from build123d import *

# Parameters (mm, degrees)
F2_R     = 1.5728770132
F3_DEPTH = 20.955
F4_R     = 4.7463390005
F5_DEPTH = 9.525


# Not quite as in the source:
# - a feature names something its author has since deleted; it is built from what else it names


with BuildPart() as f1:
    # F0 (on Front) → F1 (revolve)
    with BuildSketch(Plane.XZ):
        with BuildLine():
            Line((0, 20.9652427214), (0, 6.7289513536))
            Line((0, 6.7289513536), (0, -22.2147572786))
            Line((0, -22.2147572786), (3.7280632295, -22.2147572786))
            Line((3.7280632295, -22.2147572786), (7.0464526415, -17.7902411669))
            Line((7.0464526415, -17.7902411669), (3.7280632295, -17.7902411669))
            Line((3.7280632295, -17.7902411669), (3.7280632295, -14.6562093869))
            Line((3.7280632295, -14.6562093869), (14.6050014645, -10.7847582549))
            ThreePointArc((14.6050014645, -10.7847582549), (13.3991858149, -6.7201295533), (16.2641917467, -3.5949193407))
            Line((16.2641917467, -3.5949193407), (23.8227405697, -3.5949193407))
            Line((23.8227405697, -3.5949193407), (31.75, 14.5086767152))
            Line((31.75, 14.5086767152), (14.6050014645, 14.5086767152))
            Line((14.6050014645, 14.5086767152), (8.0961844996, 14.5086767152))
            Line((8.0961844996, 14.5086767152), (8.0961844996, 20.9652427214))
            Line((8.0961844996, 20.9652427214), (0, 20.9652427214))
        make_face()
    revolve(axis=Axis((0, 0, -7.7429029625), (0, 0, -1)))

    # F2 (on face) → F3 (cut)
    with BuildSketch(Plane(origin=(0, 0, -22.2147572786), x_dir=(1, 0, 0), z_dir=(0, 0, -1))):
        Circle(F2_R)
    extrude(amount=-F3_DEPTH, mode=Mode.SUBTRACT)

    # F4 (on face) → F5 (cut)
    with BuildSketch(Plane.XY.offset(20.9652427214)):
        Circle(F4_R)
    extrude(amount=-F5_DEPTH, mode=Mode.SUBTRACT)


solid = f1.part
Design review of the part built by this model. Coordinates are the model's own, in mm. A direction names the side the tool comes from. Round coordinates to 2 decimals unless told otherwise and drop trailing zeros. Order: outer loops, then holes, each group sorted by start corner. A loop starts at its lowest first (then second) coordinate and runs counter-clockwise, first axis right, second up.
1) Consider section C-C (z = 3). State the section outline as (x, y) points.
The answers:
outline: circle Ø53.42 at (0, 0)
2) Clearance check with flat-ended pins moving along their axes: pin 1 Ø5.5 at (x, y) = (0, 0) entering from +Z; pin 2 Ø3 at (x, z) = (-20.5, 10.5) entering from -Y; pin 3 Ø3 at (y, z) = (21, 5.5) entering from +X; pin 4 Ø3.5 at (x, y) = (0, 0) entering from -Z. State where each tip first meets the part, or that it passes through.
The answers:
pin 1: stops at z = 11.44
pin 2: stops at y = -23.47
pin 3: stops at x = 20.09
pin 4: stops at z = -22.21
3) Machinability: for faces 1 (the cylindrical face through (-0.485, -3.696, -16.201)), 2 (the flat face through (3.5, 3.5, 20.965)), 3 (the flat face through (0, 0, -1.26)), 4 (the flat face through (0, 2, -22.215)), 5 (the flat face through (7, 7, 14.509)), which of the approach directions +Z, -Z, +X, -X, +Y, -Y give a long, thin tool a straight path to every point of the face, cutting with its end or side? Answer none if there is none.
The answers:
face 1: none
face 2: +Z, +X, -X, +Y, -Y
face 3: -Z
face 4: -Z, +X, -X, +Y, -Y
face 5: +Z
4) For L1, parallel to Y at x = 0, z = 18.25; L2, parallel to X at y = 0, z = -17; L3, parallel to Z at x = -7, y = -17.5, list the stretches that pass through material, from the lowest coordinate up.
The answers:
L1: y = -8.1 to -4.75, 4.75 to 8.1
L2: x = -3.73 to -1.57, 1.57 to 3.73
L3: z = -3.59 to 14.51
5) Draft analysis for pull direction X (two halves, no side actions). For faces 6 (the conical face through (-5.27, 23.74, -2.46)), 7 (the cylindrical face through (-0.618, 4.706, 16.269)), 8 (the flat face through (-16, 5, -3.595)), state which applies: released by +X, released by -X, zero draft, split by the parting line, or undercut.
The answers:
face 6: split by the parting line
face 7: undercut
face 8: zero draft
6) Consider section A-A (x = 0). State the section outline as (y, z) points (3 decimals), plus the area to 3 significant figures.
The answers:
outline: (-31.75, 14.509) - (-23.823, -3.595) - (-16.264, -3.595) arc R4.303 cw to (-14.605, -10.785) - (-3.728, -14.656) - (-3.728, -17.79) - (-7.046, -17.79) - (-3.728, -22.215) - (-1.573, -22.215) - (-1.573, -1.26) - (1.573, -1.26) - (1.573, -22.215) - (3.728, -22.215) - (7.046, -17.79) - (3.728, -17.79) - (3.728, -14.656) - (14.605, -10.785) arc R4.303 cw to (16.264, -3.595) - (23.823, -3.595) - (31.75, 14.509) - (8.096, 14.509) - (8.096, 20.965) - (4.746, 20.965) - (4.746, 11.44) - (-4.746, 11.44) - (-4.746, 20.965) - (-8.096, 20.965) - (-8.096, 14.509) - close
area: 1,300 mm2
